Source: CAD feature listing. Evaluate the final solid. Frame: model axes, mm. Give positions to 0.01 mm unless a question says otherwise; leave off trailing zeros. Order: outer loops, then holes, each group sorted by start corner. A loop starts at its lowest first (then second) coordinate and runs counter-clockwise, first axis right, second up. Notation, with made-up numbers: (-13, 22.25) -> (27, 22.25) arc R20 ccw to (27, 32.25) -> close; hole circle Ø11 at (65.25, -14). An arc over 180 degrees is marked (long way). Use CSV: the item, a comma, the result in double quotes.
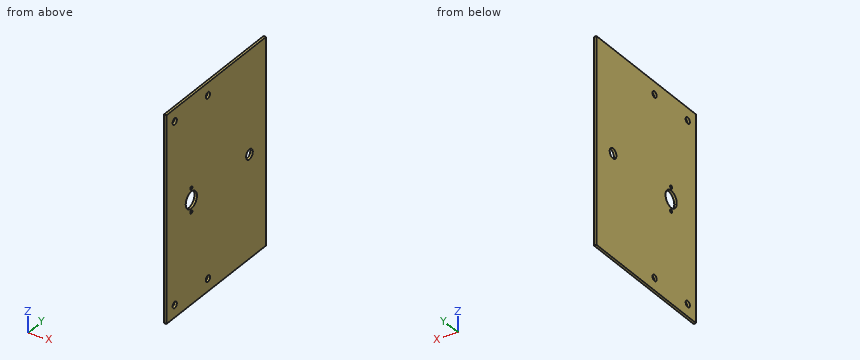
Autodesk Inventor part; units mm, degrees
ref_plane "YZ Plane" through (0, 0, 0) normal (1, 0, 0) x (0, 1, 0)
ref_plane "XZ Plane" through (0, 0, 0) normal (0, 1, 0) x (-1, 0, 0)
ref_plane "XY Plane" through (0, 0, 0) normal (0, 0, 1) x (1, 0, 0)
sketch "Skizze1" plane through (0, 0, 0) normal (1, 0, 0) x (0, 1, 0)
  line L0 (-30, 82.5) -> (30, 82.5)
  line L1 (30, 82.5) -> (30, -82.5)
  line L2 (30, -82.5) -> (-30, -82.5)
  line L3 (-30, -82.5) -> (-30, 82.5)
  line L4 (-30, 82.5) -> (30, -82.5) construction
  line L5 (30, 82.5) -> (-30, -82.5) construction
  point P0 (0, 0)
  dimension "d0" = 165
  dimension "d1" = 60
extrude "Extrusion1" add sketch "Skizze1" along normal blind 2
sketch "Skizze2" plane through (2, 0, 0) normal (1, 0, 0) x (0, 0, -1)
  circle A0 centre (0, 0) radius 6.75
  circle A1 centre (9.5, 0) radius 1.25
  circle A2 centre (-9.5, 0) radius 1.25
  circle A3 centre (-72.5, 20) radius 2.5
  circle A4 centre (-72.5, -20) radius 2.5
  circle A5 centre (72.5, 20) radius 2.5
  circle A6 centre (72.5, -20) radius 2.5
  line L0 (-82.5, 30) -> (-82.5, -30)
  line L1 (-82.5, -30) -> (82.5, -30)
  line L2 (82.5, 30) -> (-82.5, 30)
  dimension "d4" = 13.5
  dimension "d5" = 19
  dimension "d6" = 9.5
  dimension "d7" = 2.5
  dimension "d8" = 2.5
  dimension "d9" = 5
  dimension "d10" = 5
  dimension "d11" = 5
  dimension "d12" = 5
  dimension "d14" = 145
  dimension "d15" = 72.5
  dimension "d16" = 145
  dimension "d17" = 72.5
  dimension "d18" = 10
  dimension "d19" = 10
  dimension "d20" = 10
  dimension "d21" = 10
extrude "Extrusion2" cut sketch "Skizze2" against normal blind 5
sketch "Skizze3" plane through (0, 30, 82.5) normal (0, 1, 0) x (1, 0, 0)
  line L0 (0, 165) -> (0, 0)
  line L1 (0, 0) -> (2, 0)
  line L2 (2, 0) -> (2, 165)
  line L3 (2, 165) -> (0, 165)
  line L4 (0, 165) -> (0, 0)
  point P0 (0, 82.5)
extrude "Extrusion3" add sketch "Skizze3" along normal blind 60
sketch "Skizze4" plane through (2, 0, 0) normal (1, 0, 0) x (0, 0, -1)
  circle A0 centre (0, 70) radius 4
  point P0 (0, 0)
  dimension "d26" = 70
  dimension "d27" = 8
extrude "Extrusion4" cut sketch "Skizze4" against normal blind 45
equation "\"d22\" = d11"
properties part number "Motorblechdive"
1. Ray query, line 1 along Y through (x, z) = (0.9, -72.5); line 2 along Y through (x, z) = (1.4, 0); line 3 along Y through (x, z) = (1, 9.5). Return the intervals inside material, ascending.
Answer below:
line 1,"y = -30 to -22.5, -17.5 to 17.5, 22.5 to 90"
line 2,"y = -30 to -6.75, 6.75 to 66, 74 to 90"
line 3,"y = -30 to -1.25, 1.25 to 90"
2. Section query A-A on z = -72.5. Return loops of the section in (x, y), plus the area to 3 significant figures.
Answer below:
outline,"(0, -30) -> (2, -30) -> (2, -22.5) -> (0, -22.5) -> close; (0, -17.5) -> (2, -17.5) -> (2, 17.5) -> (0, 17.5) -> close; (0, 22.5) -> (2, 22.5) -> (2, 90) -> (0, 90) -> close"
area,"220 mm²"
3. Section query B-B on y = 20. Return loops of the section in (x, z).
Answer below:
outline,"(0, -82.5) -> (2, -82.5) -> (2, -75) -> (0, -75) -> close; (0, -70) -> (2, -70) -> (2, 70) -> (0, 70) -> close; (0, 75) -> (2, 75) -> (2, 82.5) -> (0, 82.5) -> close"
